For this review, take the finished solid that the model builds, in its own axes (mm). Face numbers are marked on the shaded views. A direction names the side the tool comes from. Round coordinates to 2 decimals unless told otherwise and drop trailing zeros. Write each loop counter-clockwise with the first axis right and the second up, starting at its lowest first coordinate (ties: lowest second). Pieces come first, ordered by that corner, then holes. Notation, with made-up numbers: (13, 12.25) - (19, 12.25) arc R21 ccw to (19, 42.25) - close; hole circle Ø9 at (-10, -37.75). An arc over 180 degrees is marked (long way). One line per item, written item: value. Start each with the question number.
Q1. Clearance check with flat-ended pins moving along their axes: pin 1 Ø0.9 at (x, z) = (27.5, 1.5) entering from +Y; pin 2 Ø5 at (x, y) = (-5.5, 7.5) entering from +Z; pin 3 Ø2 at (x, z) = (-2.5, 5) entering from -Y; pin 4 Ø2 at (x, y) = (0, -7) entering from +Z. State where each tip first meets the part, or that it passes through.
Q2. Tool access review of the marked faces 4 and 5: name each direction out of +Z, -Z, +X, -X, +Y, -Y from which nothing blocks a thin tool from reaching the whole face with its end or side.
Q3. Add section D-D on z = 7.75. Write out the cut boundary in (x, y), and give its area (3 significant figures).
Q4. Add section B-B on x = 0. Write out the cut boundary in (y, z).
Q5. Add section A-A on y = 0. Write out the cut boundary in (x, z).
Q6. Mouldability with a two-part tool opening along X and no side actions: class the marked faces 1, 2 and 3 as +X half, -X half, draft (parallel to the pull), parting line (faces both ways), or undercut.
Q7. Add section C-C on z = 2.25. Write out the cut boundary in (x, y), and give its area (3 significant figures).
Q8. For probe 1 along Y at (x, z) = (0, 1.65); probe 2 along Z at (x, y) = (2, 1); probe 3 along Y at (x, z) = (35, 2.35), list the stretches that pass through material, from the lowest coordinate up.
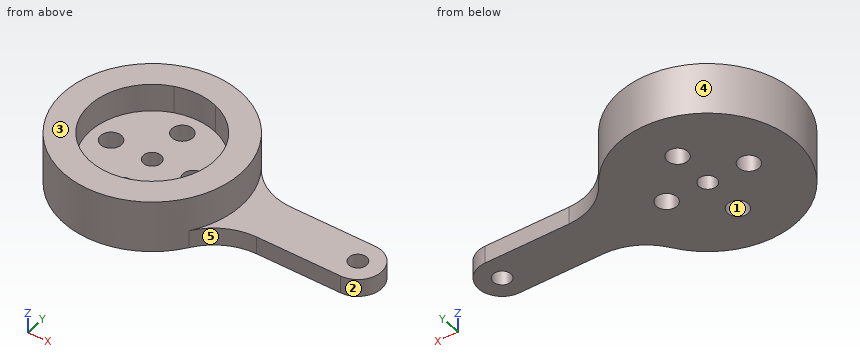
```python
from build123d import *
from build123d.topology import SkipClean

# Parameters (mm, degrees)
SKETCH1_R           = 15
BOSS_EXTRUDE1_DEPTH = 8.8
CUT_EXTRUDE1_DEPTH  = 5
SKETCH3_R           = 1.5
CUT_EXTRUDE2_DEPTH  = 5
BOSS_EXTRUDE2_DEPTH = 3
FILLET1_R           = 10
FILLET2_R           = 10
SKETCH6_R           = 1.5
CUT_EXTRUDE4_DEPTH  = 3
SKETCH7_R           = 10.5
CUT_EXTRUDE6_DEPTH  = 5
BOSS_EXTRUDE3_DEPTH = 0.3
BOSS_EXTRUDE4_START = -4.7
BOSS_EXTRUDE4_DEPTH = 4.7
SKETCH11_R          = 1.5
CUT_EXTRUDE7_DEPTH  = 43.083250825
SKETCH12_R          = 1.75
CUT_EXTRUDE8_DEPTH  = 43.701756404


with BuildPart() as part:
    # Sketch1 → Boss-Extrude1 (new body)
    with BuildSketch(Plane.XY):
        Circle(SKETCH1_R)
    extrude(amount=BOSS_EXTRUDE1_DEPTH)

    # Sketch2 → Cut-Extrude1 (cut)
    with BuildSketch(Plane.XY.offset(8.8)):
        with BuildLine():
            Line((-2.469689731, 16.888114198), (-4.5, 3.968626967))
            ThreePointArc((-4.5, 3.968626967), (-6, 0), (-4.5, -3.968626967))
            Line((-4.5, -3.968626967), (-2.469689731, -16.888114198))
            ThreePointArc((-2.469689731, -16.888114198), (0, -19), (2.469689731, -16.888114198))
            Line((2.469689731, -16.888114198), (4.5, -3.968626967))
            ThreePointArc((4.5, -3.968626967), (6, 0), (4.5, 3.968626967))
            Line((4.5, 3.968626967), (2.469689731, 16.888114198))
            ThreePointArc((2.469689731, 16.888114198), (0, 19), (-2.469689731, 16.888114198))
        make_face()
    extrude(amount=-CUT_EXTRUDE1_DEPTH, mode=Mode.SUBTRACT)

    # Sketch3 → Cut-Extrude2 (cut)
    with BuildSketch(Plane.XY.offset(3.8)):
        Circle(SKETCH3_R)
    extrude(amount=-CUT_EXTRUDE2_DEPTH, mode=Mode.SUBTRACT)

    # Sketch4 → Boss-Extrude2 (add)
    with BuildSketch(Plane(origin=(0, 0, 0), x_dir=(-1, 0, 0), z_dir=(0, 0, -1))):
        with BuildLine():
            Line((-35, 4), (-14.456832295, 4))
            ThreePointArc((-14.456832295, 4), (-15, 0), (-14.456832295, -4))
            Line((-14.456832295, -4), (-35, -4))
            ThreePointArc((-35, -4), (-39, 0), (-35, 4))
        make_face()
    extrude(amount=-BOSS_EXTRUDE2_DEPTH)

    # Fillet1
    fillet1_edges = [part.edges().sort_by_distance(p)[0] for p in [
        (14.456832295, 4, 1.5),
    ]]
    fillet(fillet1_edges, radius=FILLET1_R)

    # Fillet2
    fillet2_edges = [part.edges().sort_by_distance(p)[0] for p in [
        (14.456832295, -4, 1.5),
    ]]
    fillet(fillet2_edges, radius=FILLET2_R)

    # Sketch6 → Cut-Extrude4 (cut)
    with BuildSketch(Plane.XY.offset(3)):
        with Locations((35, 0)):
            Circle(SKETCH6_R)
    extrude(amount=-CUT_EXTRUDE4_DEPTH, mode=Mode.SUBTRACT)

    # Sketch7 → Cut-Extrude6 (cut)
    with BuildSketch(Plane.XY.offset(3.8)):
        Circle(SKETCH7_R)
    extrude(amount=CUT_EXTRUDE6_DEPTH, mode=Mode.SUBTRACT)

    # Sketch8 → Boss-Extrude3 (add)
    with BuildSketch(Plane.XY.offset(3.8)):
        with BuildLine():
            Line((-2.808083405, 14.73481142), (-3.572005324, 9.873741842))
            ThreePointArc((-3.572005324, 9.873741842), (-10.5, 0), (-3.572005324, -9.873741842))
            Line((-3.572005324, -9.873741842), (-2.808083405, -14.73481142))
            ThreePointArc((-2.808083405, -14.73481142), (0, -15), (2.808083405, -14.73481142))
            Line((2.808083405, -14.73481142), (3.572005324, -9.873741842))
            ThreePointArc((3.572005324, -9.873741842), (10.5, 0), (3.572005324, 9.873741842))
            Line((3.572005324, 9.873741842), (2.808083405, 14.73481142))
            ThreePointArc((2.808083405, 14.73481142), (0, 15), (-2.808083405, 14.73481142))
        make_face()
    extrude(amount=BOSS_EXTRUDE3_DEPTH)

    # Sketch9 → Boss-Extrude4 (add)
    with SkipClean():  # the faces are left unmerged after this step: merging them gives an invalid solid
        with BuildSketch(Plane.XY.offset(8.8).offset(BOSS_EXTRUDE4_START)):
            with BuildLine():
                Line((-2.808083405, 14.73481142), (-3.572005324, 9.873741842))
                ThreePointArc((-3.572005324, 9.873741842), (0, 10.5), (3.572005324, 9.873741842))
                Line((3.572005324, 9.873741842), (2.808083405, 14.73481142))
                ThreePointArc((2.808083405, 14.73481142), (0, 15), (-2.808083405, 14.73481142))
            make_face()
            with BuildLine():
                Line((-3.572005324, -9.873741842), (-2.808083405, -14.73481142))
                ThreePointArc((-2.808083405, -14.73481142), (0, -15), (2.808083405, -14.73481142))
                Line((2.808083405, -14.73481142), (3.572005324, -9.873741842))
                ThreePointArc((3.572005324, -9.873741842), (0, -10.5), (-3.572005324, -9.873741842))
            make_face()
        extrude(amount=BOSS_EXTRUDE4_DEPTH)

    # Sketch11 → Cut-Extrude7 (cut, through all)
    with SkipClean():  # the faces are left unmerged after this step: merging them gives an invalid solid
        with BuildSketch(Plane(origin=(0, 0, 3.8), x_dir=(-1, 0, 0), z_dir=(0, 0, -1))):
            with Locations(Location((0, 0, 0), (0, 0, 180))):
                Circle(SKETCH11_R)
        extrude(amount=-CUT_EXTRUDE7_DEPTH, mode=Mode.SUBTRACT)

    # Sketch12 → Cut-Extrude8 (cut, through all)
    with SkipClean():  # the faces are left unmerged after this step: merging them gives an invalid solid
        with BuildSketch(Plane(origin=(0, 0, 0), x_dir=(-1, 0, 0), z_dir=(0, 0, -1))):
            with Locations((0, -7)):
                Circle(SKETCH12_R)
            with Locations((-7, 0)):
                Circle(SKETCH12_R)
            with Locations(Location((7, 0, 0), (0, 0, 180))):
                Circle(SKETCH12_R)
            with Locations(Location((0, 7, 0), (0, 0, 180))):
                Circle(SKETCH12_R)
        extrude(amount=-CUT_EXTRUDE8_DEPTH, mode=Mode.SUBTRACT)


solid = part.part
```
Result set:
1. pin 1: stops at y = 4
1. pin 2: stops at z = 8.8
1. pin 3: stops at y = -14.92
1. pin 4: passes through
2. face 4: +Z
2. face 5: +Z, -Z, +X, -Y
3. outline: circle Ø30 at (0, 0); hole circle Ø21 at (0, 0)
3. area: 360 mm^2
4. outline: (-15, 0) - (-8.75, 0) - (-8.75, 4.1) - (-10.5, 4.1) - (-10.5, 8.8) - (-15, 8.8) - close; (-5.25, 0) - (-1.5, 0) - (-1.5, 4.1) - (-5.25, 4.1) - close; (1.5, 0) - (5.25, 0) - (5.25, 4.1) - (1.5, 4.1) - close; (8.75, 0) - (15, 0) - (15, 8.8) - (10.5, 8.8) - (10.5, 4.1) - (8.75, 4.1) - close
5. outline: (-15, 0) - (-8.75, 0) - (-8.75, 4.1) - (-10.5, 4.1) - (-10.5, 8.8) - (-15, 8.8) - close; (-5.25, 0) - (-1.5, 0) - (-1.5, 4.1) - (-5.25, 4.1) - close; (1.5, 0) - (5.25, 0) - (5.25, 4.1) - (1.5, 4.1) - close; (8.75, 0) - (33.5, 0) - (33.5, 3) - (15, 3) - (15, 8.8) - (10.5, 8.8) - (10.5, 4.1) - (8.75, 4.1) - close; (36.5, 0) - (39, 0) - (39, 3) - (36.5, 3) - close
6. face 1: undercut
6. face 2: +X half
6. face 3: draft
7. outline: (12.43, -8.4) arc R10 cw to (20.71, -4) - (35, -4) arc R4 ccw to (35, 4) - (20.71, 4) arc R10 cw to (12.43, 8.4) arc R15 ccw (long way) to start; hole circle Ø3.5 at (-7, 0); hole circle Ø3.5 at (0, -7); hole circle Ø3.5 at (0, 7); hole circle Ø3 at (0, 0); hole circle Ø3.5 at (7, 0); hole circle Ø3 at (35, 0)
7. area: 852 mm^2
8. probe 1: y = -15 to -8.75, -5.25 to -1.5, 1.5 to 5.25, 8.75 to 15
8. probe 2: z = 0 to 4.1
8. probe 3: y = -4 to -1.5, 1.5 to 4
